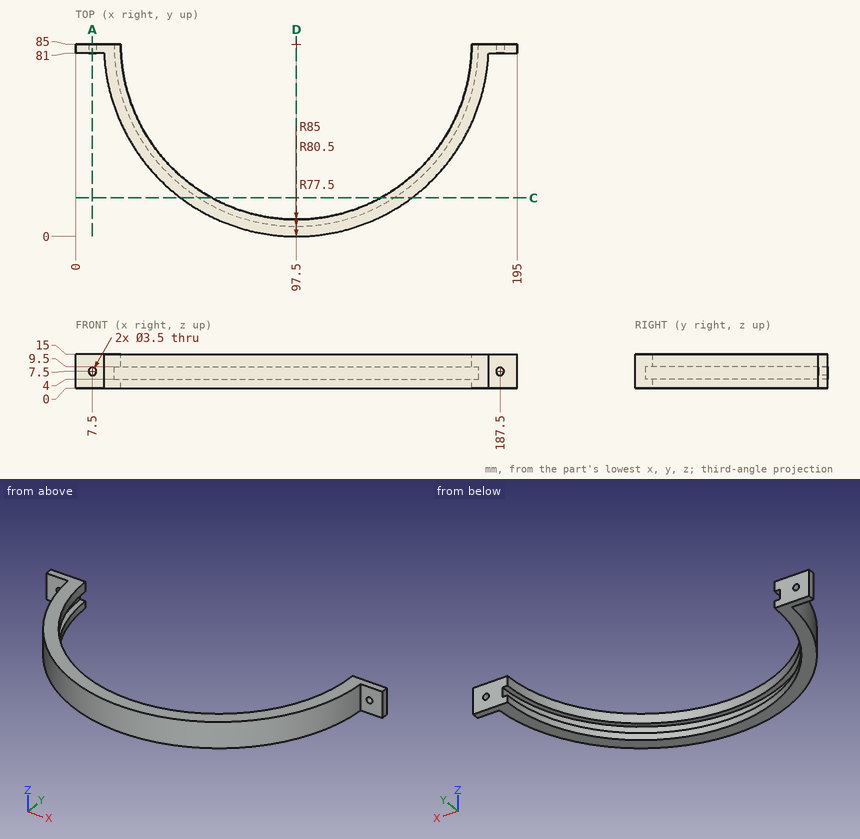
Part print with two shaded views. Sizes in mm from the minimum x, y, z corner. Coordinates: 2 decimals unless noted, no trailing zeros. Loops run counter-clockwise (first coordinate to the right, second up) from the corner with the lowest first, then second, coordinate; pieces in that order, holes last. Notation, with made-up numbers: M 55.25,-14 L 87.25,-14 A6 ccw 87.25,-9 Z; hole C 23.25,38.5 d8. An arc over 180 degrees is marked long. Use CSV: the item, a comma, the result in double quotes. Start each with the question number.
1. Flat gauge pins, fed straight in: pin 1 (4.5 mm diameter, centred on x = 7.5, z = 7.5, fed in from -Y); pin 2 (1 mm diameter, centred on x = 138, z = 7.5, fed in from +Y); pin 3 (4.5 mm diameter, centred on x = 187.5, z = 7.5, fed in from +Y); pin 4 (8 mm diameter, centred on x = 58, z = 1.5, fed in from -Y). Where does each tip first touch, or does it go through?
2. Band-saw the part on C-C, the plane y = 17. List the corners of the cut face in (x, z), then the cut area to 3 significant figures.
3. Band-saw the part on A-A, the plane x = 7.5. List the corners of the cut face in (y, z), then the cut area to 3 significant figures.
4. Band-saw the part on D-D, the plane x = 97.5. List the corners of the cut face in (y, z), then the cut area to 3 significant figures.
5. Probe probe 1 along X at (y, z) = (83.5, 7.5); probe 2 along X at (y, z) = (81.8, 7.5); probe 3 along X at (y, z) = (54.5, 4.75). List the from-to ranges inside material, lowest first. Write a range as [from, to].
Entries:
1,pin 1,"stops at y = 81"
1,pin 2,"stops at y = 15.72"
1,pin 3,"stops at y = 85"
1,pin 4,"stops at y = 7.77"
2,outline,"M 46.5,0 L 60.32,0 L 60.32,4 L 54.42,4 L 54.42,9.5 L 60.32,9.5 L 60.32,15 L 46.5,15 Z; M 134.68,0 L 148.5,0 L 148.5,15 L 134.68,15 L 134.68,9.5 L 140.58,9.5 L 140.58,4 L 134.68,4 Z"
2,area,"350 mm2"
3,outline,"M 81,0 L 85,0 L 85,5.75 L 81,5.75 Z; M 81,9.25 L 85,9.25 L 85,15 L 81,15 Z"
3,area,"46.0 mm2"
4,outline,"M 0,0 L 7.5,0 L 7.5,4 L 4.5,4 L 4.5,9.5 L 7.5,9.5 L 7.5,15 L 0,15 Z"
4,area,"96.0 mm2"
5,probe 1,"x = [0, 5.75], [9.25, 17.01], [177.99, 185.75], [189.25, 195]"
5,probe 2,"x = [0, 5.75], [9.25, 17.06], [177.94, 185.75], [189.25, 195]"
5,probe 3,"x = [18.16, 23], [172, 176.84]"
